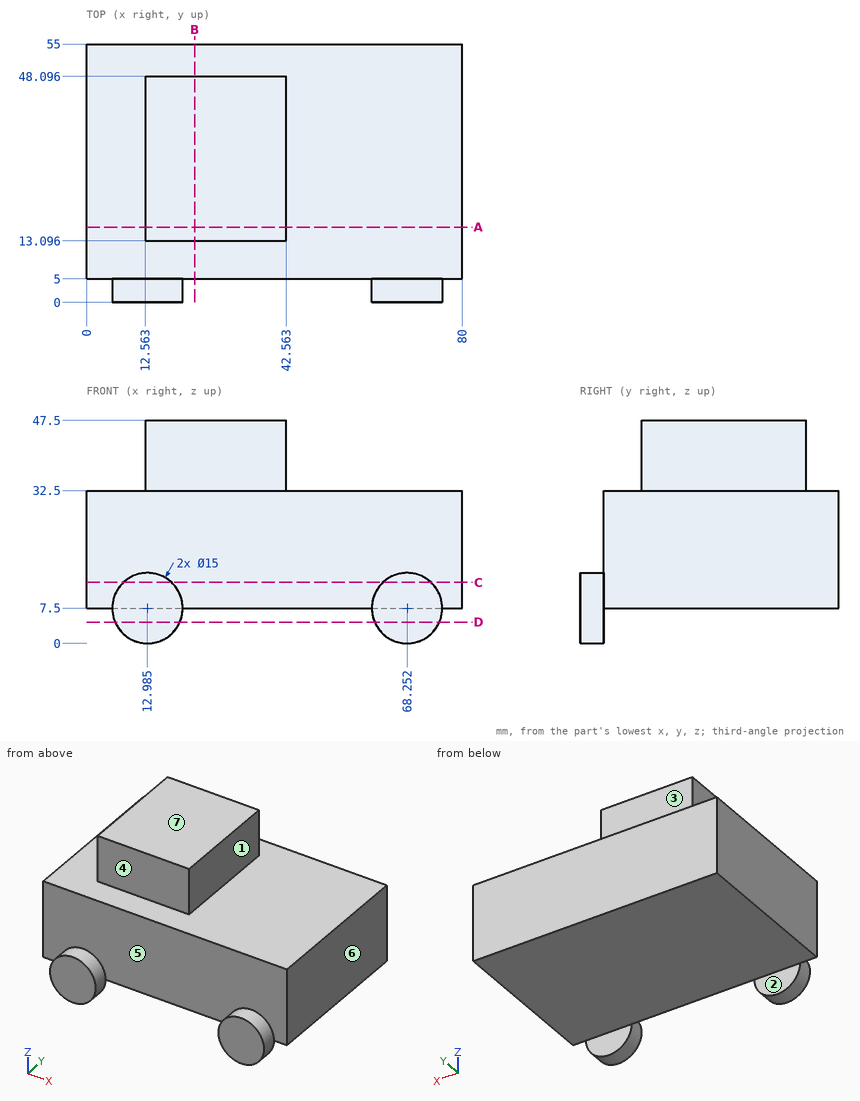
Here's the drawing with two shaded views (mm, measured from the low corner). I have some questions. A direction names the side the tool comes from. Give positions to 0.01 mm unless a question says otherwise; leave off trailing zeros. Order: outer loops, then holes, each group sorted by start corner. A loop starts at its lowest first (then second) coordinate and runs counter-clockwise, first axis right, second up. Notation, with made-up numbers: (21.5, 26) -> (43.5, 26) arc R27 ccw to (43.5, 50) -> close; hole circle Ø11 at (-8, 28). An arc over 180 degrees is marked (long way). One line per item, written item: value. Start each with the question number.
1. Imagine slicing it at A-A, the plane y = 16. List the corners of the cut face in (x, z) for me.
2. We'd pull the mould along X, two halves only. Please class the marked faces 5, 6 and 7: released by +X, released by -X, zero draft, split by the parting line, or undercut.
3. I need wall thicknesses on probe 1 along Z at (x, y) = (4.5, 43.5); probe 2 along Y at (x, z) = (76.5, 8); probe 3 along Z at (x, y) = (20.5, 43). Which ranges of each line are inside material? Lowest first, please. Write a range as from..to.
4. Imagine slicing it at D-D, the plane z = 4.5. List the corners of the cut face in (x, y) for me.
5. Imagine slicing it at B-B, the plane x = 23. List the corners of the cut face in (y, z) for me, plus the area to 4 significant figures.
6. Will these pins go through, and if not, where does the flat tip stop? pin 1 Ø12 at (x, z) = (54.5, 26.5) entering from -Y; pin 2 Ø8 at (x, y) = (67, 17) entering from +Z; pin 3 Ø4 at (x, y) = (26.5, 45) entering from -Z.
7. For the marked faces 1, 2, 3 and 4, which set-ups out of +Z, -Z, +X, -X, +Y, -Y let a thin tool reach every point of the face, with its end or its side?
8. Imagine slicing it at C-C, the plane z = 13. List the corners of the cut face in (x, y) for me, plus the area to 3 significant figures.
Values follow:
1. outline: (0, 7.5) -> (80, 7.5) -> (80, 32.5) -> (42.56, 32.5) -> (42.56, 47.5) -> (12.56, 47.5) -> (12.56, 32.5) -> (0, 32.5) -> close
2. face 5: undercut
2. face 6: released by +X
2. face 7: zero draft
3. probe 1: z = 7.5..32.5
3. probe 2: y = 5..55
3. probe 3: z = 7.5..47.5
4. outline: (6.11, 0) -> (19.86, 0) -> (19.86, 5) -> (6.11, 5) -> close; (61.38, 0) -> (75.13, 0) -> (75.13, 5) -> (61.38, 5) -> close
5. outline: (5, 7.5) -> (55, 7.5) -> (55, 32.5) -> (48.1, 32.5) -> (48.1, 47.5) -> (13.1, 47.5) -> (13.1, 32.5) -> (5, 32.5) -> close
5. area: 1,775 mm2
6. pin 1: stops at y = 5
6. pin 2: stops at z = 32.5
6. pin 3: stops at z = 7.5
7. face 1: +Z, +X, +Y, -Y
7. face 2: -Z, +X, -X, +Y
7. face 3: +Z, +X, -X, +Y
7. face 4: +Z, +X, -X, -Y
8. outline: (0, 5) -> (7.89, 5) -> (7.89, 0) -> (18.08, 0) -> (18.08, 5) -> (63.15, 5) -> (63.15, 0) -> (73.35, 0) -> (73.35, 5) -> (80, 5) -> (80, 55) -> (0, 55) -> close
8. area: 4,100 mm2
